```python
from build123d import *

# Parameters (mm, degrees)
F0_W     = 42
F0_H     = 42
F1_DEPTH = 10
F2_SIZE  = 4
F3_R     = 2
F5_DEPTH = 3
F6_R     = 1.5
F7_DEPTH = 10.001
F8_R     = 4.5
F9_DEPTH = 10.001


with BuildPart() as f1:
    # F0 (on Front) → F1 (new body)
    with BuildSketch(Plane.XZ):
        Rectangle(F0_W, F0_H)
    extrude(amount=F1_DEPTH)

    # F2
    f2_edges = [f1.edges().sort_by_distance(p)[0] for p in [
        (-21, -5, 21),
        (21, -5, 21),
        (21, -5, -21),
        (-21, -5, -21),
    ]]
    chamfer(f2_edges, length=F2_SIZE)

    # F3
    f3_edges = [f1.edges().sort_by_distance(p)[0] for p in [
        (-17, -5, 21),
        (17, -5, 21),
        (21, -5, 17),
        (21, -5, -17),
        (17, -5, -21),
        (-17, -5, -21),
        (-21, -5, -17),
        (-21, -5, 17),
    ]]
    fillet(f3_edges, radius=F3_R)

    # F4 (on face) → F5 (cut)
    with BuildSketch(Plane(origin=(0, 0, 0), x_dir=(-1, 0, 0), z_dir=(0, 1, 0))):
        with BuildLine():
            ThreePointArc((-14.5105618091, 21), (-17.8908729653, 17.8908729653), (-21, 14.5105618091))
            Line((-21, 14.5105618091), (-21, -14.5105618091))
            ThreePointArc((-21, -14.5105618091), (-17.8908729653, -17.8908729653), (-14.5105618091, -21))
            Line((-14.5105618091, -21), (14.5105618091, -21))
            ThreePointArc((14.5105618091, -21), (17.8908729653, -17.8908729653), (21, -14.5105618091))
            Line((21, -14.5105618091), (21, 14.5105618091))
            ThreePointArc((21, 14.5105618091), (17.8908729653, 17.8908729653), (14.5105618091, 21))
            Line((14.5105618091, 21), (-14.5105618091, 21))
        make_face()
    extrude(amount=-F5_DEPTH, mode=Mode.SUBTRACT)

    # F6 (on face) → F7 (cut, through all)
    with BuildSketch(Plane.XZ.offset(10)):
        with Locations((-15.5, 15.5)):
            Circle(F6_R)
        with Locations((-15.5, -15.5)):
            Circle(F6_R)
        with Locations((15.5, -15.5)):
            Circle(F6_R)
        with Locations((15.5, 15.5)):
            Circle(F6_R)
    extrude(amount=-F7_DEPTH, mode=Mode.SUBTRACT)

    # F8 (on face) → F9 (cut, through all)
    with BuildSketch(Plane.XZ.offset(10)):
        Circle(F8_R)
    extrude(amount=-F9_DEPTH, mode=Mode.SUBTRACT)


solid = f1.part
```
The model under review builds one solid part; all positions refer to its coordinate system, in mm. A direction names the side the tool comes from. Coordinates: 2 decimals unless noted, no trailing zeros. Loops run counter-clockwise (first coordinate to the right, second up) from the corner with the lowest first, then second, coordinate; pieces in that order, holes last. Notation, with made-up numbers: (32, -28.75) -> (86, -28.75) arc R5 ccw to (86, -23.75) -> close; hole circle Ø6 at (0, 85.5). An arc over 180 degrees is marked (long way). Answer as CSV lines item,"result".
Item 1: Insertion check: pin 1 (2.5 mm diameter, centred on x = 15.5, z = -15.5, fed in from +Y); pin 2 (12 mm diameter, centred on x = -16.5, z = -1, fed in from +Y). Each pin has a flat end and moves straight along its axis. Give the tip position at first contact, or say it passes through.
Results below:
pin 1,"passes through"
pin 2,"stops at y = -3"
Item 2: Draft analysis for pull direction Z (two halves, no side actions). For faces 1 (the cylindrical face through (-17, -6.55, -15.43)), 2 (the flat face through (18, 0, 18)), 3 (the flat face through (19, -5, 19)), state which applies: +Z half, -Z half, draft (parallel to the pull), parting line (faces both ways), or undercut.
Results below:
face 1,"undercut"
face 2,"draft"
face 3,"+Z half"
Item 3: Take a section at D-D, the plane y = -6.75. State the section outline as (x, z) points, and give its area (3 significant figures).
Results below:
outline,"(-21, -16.17) arc R2 ccw to (-20.41, -17.59) -> (-17.59, -20.41) arc R2 ccw to (-16.17, -21) -> (16.17, -21) arc R2 ccw to (17.59, -20.41) -> (20.41, -17.59) arc R2 ccw to (21, -16.17) -> (21, 16.17) arc R2 ccw to (20.41, 17.59) -> (17.59, 20.41) arc R2 ccw to (16.17, 21) -> (-16.17, 21) arc R2 ccw to (-17.59, 20.41) -> (-20.41, 17.59) arc R2 ccw to (-21, 16.17) -> close; hole circle Ø3 at (-15.5, -15.5); hole circle Ø3 at (-15.5, 15.5); hole circle Ø9 at (0, 0); hole circle Ø3 at (15.5, -15.5); hole circle Ø3 at (15.5, 15.5)"
area,"1,640 mm2"
Item 4: Machinability: for faces 4 (the cylindrical face through (17.845, -1.479, 17.936)), 5 (the flat face through (-18, 0, -18)), which of the approach directions +Z, -Z, +X, -X, +Y, -Y give a long, thin tool a straight path to every point of the face, cutting with its end or side? Answer none if there is none.
Results below:
face 4,"+Y"
face 5,"+Z, -Z, +X, -X, +Y"
Item 5: Take a section at C-C, the plane x = 0. State the section outline as (y, z) points, and give its area (3 significant figures).
Results below:
outline,"(-10, -21) -> (-3, -21) -> (-3, -4.5) -> (-10, -4.5) -> close; (-10, 4.5) -> (-3, 4.5) -> (-3, 21) -> (-10, 21) -> close"
area,"231 mm2"
Item 6: For L1, parallel to Z at x = -15.5, y = -8; L2, parallel to Y at x = 5, z = 16.5; L3, parallel to X at y = -2, z = 16.5, list the stretches that pass through material, from the lowest coordinate up.
Results below:
L1,"z = -21 to -17, -14 to 14, 17 to 21"
L2,"y = -10 to -3"
L3,"x = -20.97 to -19.23, 19.23 to 20.97"
Item 7: Take a section at A-A, the plane x = -15.5. State the section outline as (y, z) points.
Results below:
outline,"(-10, -21) -> (0, -21) -> (0, -20.14) -> (-3, -20.14) -> (-3, -17) -> (-10, -17) -> close; (-10, -14) -> (-3, -14) -> (-3, 14) -> (-10, 14) -> close; (-10, 17) -> (-3, 17) -> (-3, 20.14) -> (0, 20.14) -> (0, 21) -> (-10, 21) -> close"
Item 8: Take a section at B-B, the plane y = -2.5. State the section outline as (x, z) points, and give its area (3 significant figures).
Results below:
outline,"(-21, -16.17) arc R2 ccw to (-20.41, -17.59) -> (-17.59, -20.41) arc R2 ccw to (-16.17, -21) -> (-14.51, -21) arc R55 cw to (-21, -14.51) -> close; (-21, 14.51) arc R55 cw to (-14.51, 21) -> (-16.17, 21) arc R2 ccw to (-17.59, 20.41) -> (-20.41, 17.59) arc R2 ccw to (-21, 16.17) -> close; (14.51, -21) -> (16.17, -21) arc R2 ccw to (17.59, -20.41) -> (20.41, -17.59) arc R2 ccw to (21, -16.17) -> (21, -14.51) arc R55 cw to start; (14.51, 21) arc R55 cw to (21, 14.51) -> (21, 16.17) arc R2 ccw to (20.41, 17.59) -> (17.59, 20.41) arc R2 ccw to (16.17, 21) -> close"
area,"46.8 mm2"
